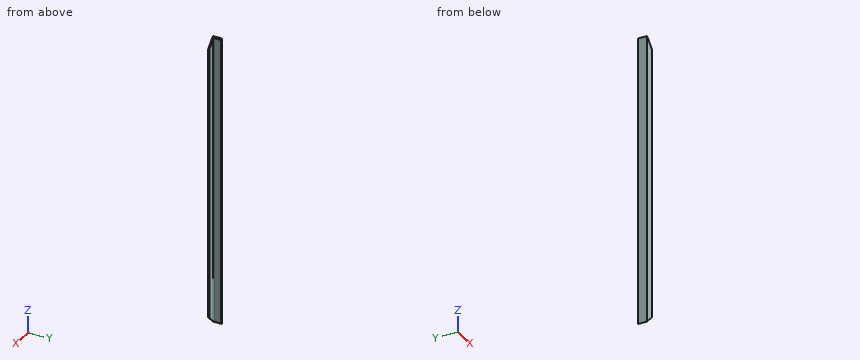
Autodesk Inventor part; units mm, degrees
ref_plane "Start plane" through (0, 0, 0) normal (0, 0, 1) x (1, 0, 0)
ref_plane "End plane" through (0, 0, 1231.9) normal (0, 0, 1) x (1, 0, 0)
ref_plane "Work Plane4" through (0, 19.05, 1231.9) normal (0.7071, 0, 0.7071) x (0.7071, 0, -0.7071)
ref_plane "Start plane" through (0, 0, 0) normal (0, 0, 1) x (1, 0, 0)
ref_plane "End plane" through (0, 0, 1231.9) normal (0, 0, 1) x (1, 0, 0)
sketch "Sketch" plane through (0, 0, 0) normal (0, 0, 1) x (1, 0, 0)
  line L0 (38.1, 0) -> (0, 0)
  line L1 (0, 0) -> (0, 38.1)
  line L2 (0, 38.1) -> (2.4765, 38.1)
  line L3 (4.7625, 35.814) -> (4.7625, 9.5885)
  line L4 (9.5885, 4.7625) -> (35.814, 4.7625)
  line L5 (38.1, 2.4765) -> (38.1, 0)
  line L6 (0, -11.0414) -> (0, 31.5385) construction
  line L7 (-11.0414, 0) -> (31.5385, 0) construction
  arc A0 (4.7625, 9.5885) -> (9.5885, 4.7625) centre (9.5885, 9.5885) ccw
  arc A1 (4.7625, 35.814) -> (2.4765, 38.1) centre (2.4765, 35.814) ccw
  arc A2 (38.1, 2.4765) -> (35.814, 4.7625) centre (35.814, 2.4765) ccw
  line L8 (0, 48.4964) -> (0, -20.9644) construction
  line L9 (-20.9644, 0) -> (48.4964, 0) construction
  point P0 (4.7625, 38.1)
  point P1 (4.7625, 4.7625)
  point P2 (38.1, 4.7625)
  dimension "d0" = 38.1
  dimension "d1" = 38.1
  dimension "d2" = 4.7625
  dimension "d3" = 4.7625
  dimension "d10" = 0
  dimension "d11" = 0
  dimension "d14" = 4.826
  dimension "d15" = 2.286
extrude "Body" add sketch "Sketch" along normal up to surface (1231.9 mm away) from surface at 0
sketch "Sketch3" plane through (0, 0, 0) normal (0, 0, 1) x (1, 0, 0)
  line L0 (0, 0) -> (10, 0)
ref_plane "Work Plane3" through (0, 0, 0) normal (0, -1, 0) x (1, 0, 0)
sketch "Sketch4" plane through (0, 0, 0) normal (0, -1, 0) x (1, 0, 0)
  line L0 (-2, 0) -> (12, 0)
  line L1 (-2, 1231.9) -> (12, 1231.9)
  dimension "d17" = 1231.9
ref_plane "Work Plane4" through (0, 19.05, 1231.9) normal (0.7071, 0, 0.7071) x (0.7071, 0, -0.7071)
split "Split1" plane through (0, 19.05, 1231.9) removes the side toward (0.7071, 0, 0.7071)
ref_plane "Work Plane5" through (0, 19.05, 0) normal (0.7071, 0, -0.7071) x (-0.7071, 0, -0.7071)
split "Split2" plane through (0, 19.05, 0) removes the side toward (0.7071, 0, -0.7071)
equation "\"d0\" = G_H"
equation "\"d1\" = G_H"
equation "\"d2\" = G_T"
equation "\"d3\" = G_T"
equation "\"d14\" = G_IR"
equation "\"d15\" = G_ER"
equation "\"d4\" = G_L"
equation "\"G_H\" = 38.1"
equation "\"G_T\" = 4.7625"
equation "\"G_ER\" = 2.286"
equation "\"G_IR\" = 4.826"
equation "\"G_L\" = d17"
equation "\"ex\" = 0"
equation "\"G_OFFSET_START\" = 0"
equation "\"G_OFFSET_END\" = 0"
equation "\"d13\" = G_OFFSET_END + B_L"
equation "\"B_L\" = 1231.9"
properties part number "AISC - L 1.5 x 1.5 x 3/16 - 48.5" material "Aluminum 6061"
For this review, take the finished solid that the model builds, in its own axes (mm). Give positions to 0.01 mm unless a question says otherwise; leave off trailing zeros. Loops run counter-clockwise (first coordinate to the right, second up) from the corner with the lowest first, then second, coordinate; pieces in that order, holes last.
Item 1: Take a section at C-C, the plane y = 24.5. State the section outline as (x, z) points.
Item 2: For line 1 along X through (y, z) = (21, 571.5); line 2 along X through (y, z) = (3, 850), list the stretches that pass through material, from the lowest coordinate up.
Item 3: Take a section at A-A, the plane z = 937.5. State the section outline as (x, y) points.
Item 4: Insertion check: pin 1 (12 mm diameter, centred on y = 21.5, z = 229.5, fed in from +X); pin 2 (1.5 mm diameter, centred on x = 23, z = 225, fed in from -Y); pin 3 (21 mm diameter, centred on x = 25, z = 793, fed in from +Y). Each pin has a flat end and moves straight along its axis. Give the tip position at first contact, or say it passes through.
Item 5: Take a section at B-B, the plane x = 21. State the section outline as (y, z) points, and give its area (3 significant figures).
Calculated:
1. outline: (0, 0) - (4.76, 4.76) - (4.76, 1227.14) - (0, 1231.9) - close
2. line 1: x = 0 to 4.76
2. line 2: x = 0 to 38.04
3. outline: (0, 0) - (38.1, 0) - (38.1, 2.48) arc R2.29 ccw to (35.81, 4.76) - (9.59, 4.76) arc R4.83 cw to (4.76, 9.59) - (4.76, 35.81) arc R2.29 ccw to (2.48, 38.1) - (0, 38.1) - close
4. pin 1: stops at x = 4.76
4. pin 2: stops at y = 0
4. pin 3: stops at y = 4.76
5. outline: (0, 21) - (4.76, 21) - (4.76, 1210.9) - (0, 1210.9) - close
5. area: 5,670 mm2
